Autodesk Inventor part; units mm, degrees
ref_plane "YZ Plane" through (0, 0, 0) normal (1, 0, 0) x (0, 1, 0)
ref_plane "XZ Plane" through (0, 0, 0) normal (0, 1, 0) x (-1, 0, 0)
ref_plane "XY Plane" through (0, 0, 0) normal (0, 0, 1) x (1, 0, 0)
ref_plane "Work Plane1" through (25.4381, 4.2054, 4.72) normal (0, 0, 1) x (0.7071, 0.7071, 0)
sketch "Sketch1" plane through (25.4381, 4.2054, 4.72) normal (0, 0, 1) x (0.7071, 0.7071, 0)
  line L0 (-20.9611, 15.0138) -> (-186.9611, 15.0138)
  line L1 (-186.9611, 15.0138) -> (-186.9611, 95.0138)
  line L2 (-186.9611, 95.0138) -> (-20.9611, 95.0138)
  line L3 (-20.9611, 95.0138) -> (-20.9611, 15.0138)
  dimension "d0" = 166
  dimension "d1" = 80
extrude "Extrusion1" add sketch "Sketch1" along normal blind 1.6
sketch "Sketch2" plane through (25.4381, 4.2054, 6.32) normal (0, 0, 1) x (0.7071, 0.7071, 0)
  point P0 (-20.9611, 15.0138)
sketch "Sketch3" plane through (25.4381, 4.2054, 6.32) normal (0, 0, 1) x (0.7071, -0.7071, 0)
  circle A0 centre (-103.5277, -22.9611) radius 1.6
  circle A1 centre (-89.0425, -28.9611) radius 1.6
  circle A2 centre (-20.9851, -28.9611) radius 1.6
  point P0 (-15.0138, -20.9611)
ref_plane "Work Plane2" through (-28.2843, 28.2843, 4.72) normal (0.7071, -0.7071, 0) x (0, 0, 1)
extrude "Extrusion2" cut sketch "Sketch3" against normal blind 10 contours A1 | A2
sketch "Sketch4" plane through (25.4381, 4.2054, 6.32) normal (0, 0, 1) x (0.7071, -0.7071, 0)
  line L0 (-15.0138, -20.9611) -> (-95.0138, -20.9611)
  line L1 (-55.0138, -20.9611) -> (-55.0138, -186.9611) construction
  line L2 (-95.0138, -186.9611) -> (-15.0138, -186.9611)
  line L3 (-57.5138, -51.8936) -> (-52.5138, -51.8936)
  line L4 (-52.5138, -51.8936) -> (-52.5138, -20.9611)
  line L5 (-52.5138, -20.9611) -> (-57.5138, -20.9611)
  line L6 (-57.5138, -20.9611) -> (-57.5138, -51.8936)
  line L7 (-57.5138, -51.8936) -> (-52.5138, -20.9611) construction
  line L8 (-52.5138, -51.8936) -> (-57.5138, -20.9611) construction
  line L9 (-52.5138, -51.8936) -> (-77.9131, -51.8936)
  line L10 (-77.9131, -51.8936) -> (-77.9131, -46.8936)
  line L11 (-77.9131, -46.8936) -> (-52.5138, -46.8936)
  line L12 (-52.5138, -46.8936) -> (-52.5138, -51.8936)
  line L13 (-74.9089, -76.3936) -> (-35.1187, -76.3936)
  line L14 (-35.1187, -76.3936) -> (-35.1187, -72.3936)
  line L15 (-35.1187, -72.3936) -> (-74.9089, -72.3936)
  line L16 (-74.9089, -72.3936) -> (-74.9089, -76.3936)
  line L17 (-74.9089, -76.3936) -> (-35.1187, -72.3936) construction
  line L18 (-35.1187, -76.3936) -> (-74.9089, -72.3936) construction
  line L19 (-35.1187, -97.3936) -> (-74.9089, -97.3936)
  line L20 (-74.9089, -101.3936) -> (-35.1187, -97.3936) construction
  line L21 (-74.9089, -101.3936) -> (-35.1187, -101.3936)
  line L22 (-35.1187, -101.3936) -> (-74.9089, -97.3936) construction
  line L23 (-74.9089, -97.3936) -> (-74.9089, -101.3936)
  line L24 (-35.1187, -101.3936) -> (-35.1187, -97.3936)
  line L25 (-35.1187, -122.3936) -> (-74.9089, -122.3936)
  line L26 (-74.9089, -126.3936) -> (-35.1187, -122.3936) construction
  line L27 (-74.9089, -126.3936) -> (-35.1187, -126.3936)
  line L28 (-35.1187, -126.3936) -> (-74.9089, -122.3936) construction
  line L29 (-74.9089, -122.3936) -> (-74.9089, -126.3936)
  line L30 (-35.1187, -126.3936) -> (-35.1187, -122.3936)
  line L31 (-35.1187, -147.3936) -> (-74.9089, -147.3936)
  line L32 (-74.9089, -151.3936) -> (-35.1187, -147.3936) construction
  line L33 (-74.9089, -151.3936) -> (-35.1187, -151.3936)
  line L34 (-35.1187, -151.3936) -> (-74.9089, -147.3936) construction
  line L35 (-74.9089, -147.3936) -> (-74.9089, -151.3936)
  line L36 (-35.1187, -151.3936) -> (-35.1187, -147.3936)
  line L37 (-35.1187, -172.3936) -> (-74.9089, -172.3936)
  line L38 (-74.9089, -176.3936) -> (-35.1187, -172.3936) construction
  line L39 (-74.9089, -176.3936) -> (-35.1187, -176.3936)
  line L40 (-35.1187, -176.3936) -> (-74.9089, -172.3936) construction
  line L41 (-74.9089, -172.3936) -> (-74.9089, -176.3936)
  line L42 (-35.1187, -176.3936) -> (-35.1187, -172.3936)
  point P0 (-55.0138, -36.4274)
  point P1 (-55.0138, -74.3936)
  point P2 (-52.5138, -49.3936)
  point P3 (-55.0138, -99.3936)
  point P4 (-55.0138, -124.3936)
  point P5 (-55.0138, -149.3936)
  point P6 (-55.0138, -174.3936)
  point P7 (-57.5138, -51.8936)
  point P8 (-57.5138, -20.9611)
  point P9 (-57.5138, -46.8936)
  dimension "d7" = 5
  dimension "d8" = 5
  dimension "d9" = 4
  dimension "d10" = 25
  dimension "d13" = 25
extrude "Extrusion3" add sketch "Sketch4" along normal blind 0.1
equation "\"d13\" = d10"
properties part number "Antenna" material "Polystyrene"
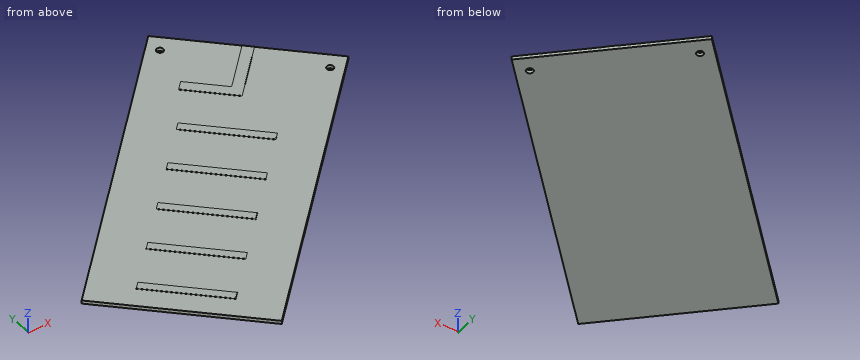
CAD build for the part. Positions are in the model's coordinates, mm. Give positions to 0.01 mm unless a question says otherwise; leave off trailing zeros. Write each loop counter-clockwise with the first axis right and the second up, starting at its lowest first coordinate (ties: lowest second). Pieces come first, ordered by that corner, then holes. Notation, with made-up numbers: (66.25, 5.5) - (115.25, 5.5) arc R30 cw to (115.25, 32.5) - close; hole circle Ø5 at (-21.5, 21.5). An arc over 180 degrees is marked (long way). Answer as CSV lines item,"result".
Q1. Flat gauge pins, fed straight in: pin 1 Ø1 at (x, z) = (-91.5, 6) entering from -Y; pin 2 Ø8 at (x, y) = (-93.5, -58.5) entering from +Z; pin 3 Ø5 at (x, y) = (-64, -2) entering from +Z. Where does each tip first touch, or does it go through?
Result set:
pin 1,"y = -92"
pin 2,"z = 6.42"
pin 3,"z = 6.32"
Q2. Band-saw the part on A-A (x = -75). Give the cut face in (y, z), and give its area (3 significant figures).
Result set:
outline,"(-75, 4.72) - (38.14, 4.72) - (38.14, 6.32) - (2.26, 6.32) - (2.26, 6.42) - (-3.39, 6.42) - (-3.39, 6.32) - (-33.09, 6.32) - (-33.09, 6.42) - (-38.75, 6.42) - (-38.75, 6.32) - (-75, 6.32) - close"
area,"182 mm²"
Q3. Band-saw the part on D-D (y = -86). Give the cut face in (x, z).
Result set:
outline,"(-148.76, 4.72) - (-86, 4.72) - (-86, 6.32) - (-128.16, 6.32) - (-128.16, 6.42) - (-133.81, 6.42) - (-133.81, 6.32) - (-148.76, 6.32) - close"
Q4. Drill centre lines: line 1 (Z direction, x = -121.5, y = -14.5); line 2 (X direction, y = -69, z = 5.7); line 3 (X direction, y = 46, z = 5.2). Where is each one in solid material? Low to high. Write a range as from..to.
Result set:
line 1,"4.72..6.32"
line 2,"-165.76..-69"
line 3,"-67.14..-59.45, -56.56..-46"
Q5. Band-saw the part on C-C (z = 5.65). Give the cut face in (x, y).
Result set:
outline,"(-173.95, -60.81) - (-117.38, -117.38) - (0, 0) - (-56.57, 56.57) - close; hole circle Ø3.2 at (-58, 46.69); hole circle Ø3.2 at (-9.88, -1.43)"
Q6. Band-saw the part on B-B (y = 16.5). Give the cut face in (x, z), and give its area (3 significant figures).
Result set:
outline,"(-96.64, 4.72) - (-16.5, 4.72) - (-16.5, 6.32) - (-36.53, 6.32) - (-36.53, 6.42) - (-43.6, 6.42) - (-43.6, 6.32) - (-53.17, 6.32) - (-53.17, 6.42) - (-60.25, 6.42) - (-60.25, 6.32) - (-96.64, 6.32) - close"
area,"130 mm²"
